```python
from build123d import *

# Parameters (mm, degrees)
CUT_EXTRUDE1_DEPTH = 4.375
CIRPATTERN1_COUNT  = 4


with BuildPart() as part:
    # Sketch1 → Revolve1 (revolve)
    with BuildSketch(Plane.XY):
        Polygon((2.1, 3), (2.1, -3), (2.6, -3), (3.125, -1.75), (2.5, -1.75), (2.5, 2.25), (3.375, 2.25), (3.375, 3), align=None)
    revolve(axis=Axis((0, 3, 0), (0, -1, 0)))

    # Sketch2 → Cut-Extrude1 (cut, symmetric)
    with BuildSketch(Plane.XY):
        Polygon((-0.249514725, 1), (0.249514725, 1), (0.625, -3), (-0.625, -3), align=None)
    cut_extrude1 = extrude(amount=CUT_EXTRUDE1_DEPTH, both=True, mode=Mode.SUBTRACT)

    # CirPattern1: Cut-Extrude1 ×4 about axis
    cirpattern1_axis = Axis((0, 3, 0), (0, 1, 0))
    for i in range(1, CIRPATTERN1_COUNT):
        add(cut_extrude1.rotate(cirpattern1_axis, i * 360 / CIRPATTERN1_COUNT), mode=Mode.SUBTRACT)


solid = part.part
```
Part model, mm, in its own coordinate system. A direction names the side the tool comes from. Round coordinates to 2 decimals unless told otherwise and drop trailing zeros. Loops run counter-clockwise (first coordinate to the right, second up) from the corner with the lowest first, then second, coordinate; pieces in that order, holes last. Notation, with made-up numbers: (-0.5, 83.5) -> (22.5, 83.5) arc R20 ccw to (22.5, 115.5) -> close; hole circle Ø7 at (18, 42.5). An arc over 180 degrees is marked (long way). Use CSV: the item, a comma, the result in double quotes. Start each with the question number.
1) Cut at B-B, the plane y = 0.5. Write the cut outline in (x, z).
2) Pull direction Y, two halves, no side cores. Call faces 1 (the flat face through (2, -1.75, -2)), 2 (the flat face through (-2, -1.75, -2)), 3 (the cylindrical face through (-0.7, 2.6, -3.3)), 4 (the flat face through (-1.6, -3, 1.7)): +Y half, -Y half, draft (parallel to the pull), parting line (faces both ways), or undercut.
3) Cut at C-C, the plane x = 0. Write the cut outline in (y, z) (3 decimals).
4) Drop flat-ended pins along their axis: P1, Ø3, axis at x = -0.5, y = -1.5, coming from the +Z side; P2, Ø3, axis at y = -2, z = 2.5, coming from the -X side; P3, Ø2, axis at x = 1.5, y = -0.5, coming from the -Z side. Give the stop position or say it passes through.
5) Cut at A-A, the plane z = 0. Write the cut outline in (x, y) (3 decimals), plus the area to 3 significant figures.
6) Which spindle directions (+Z, -Z, +X, -X, +Y, -Y) get a long thin tool onto all of the face, cutting with end or side? Do faces 5 (the cylindrical face through (2.31, 0.28, -0.96)), 6 (the flat face through (0.476, -1.416, -2.297)), 7 (the flat face through (-2.297, -1.416, -0.476)). Say none if no direction does.
7) Wall check: L1, parallel to Y at x = 2, z = -2; L2, parallel to Y at x = -2, z = 2.5; L3, parallel to X at y = -2.5, z = -0.75. Give the ranges that are in metal, low to high. Write a range as [from, to].
8) Cut at D-D, the plane y = 1.5. Write the cut outline in (x, z), plus the area to 3 significant figures.
Determined:
1,outline,"(-2.48, -0.3) arc R2.5 ccw to (-0.3, -2.48) -> (-0.3, -2.08) arc R2.1 cw to (-2.08, -0.3) -> close; (-2.48, 0.3) -> (-2.08, 0.3) arc R2.1 cw to (-0.3, 2.08) -> (-0.3, 2.48) arc R2.5 ccw to start; (0.3, -2.48) arc R2.5 ccw to (2.48, -0.3) -> (2.08, -0.3) arc R2.1 cw to (0.3, -2.08) -> close; (0.3, 2.08) arc R2.1 cw to (2.08, 0.3) -> (2.48, 0.3) arc R2.5 ccw to (0.3, 2.48) -> close"
2,face 1,"undercut"
2,face 2,"undercut"
2,face 3,"draft"
2,face 4,"-Y half"
3,outline,"(1, -2.5) -> (2.25, -2.5) -> (2.25, -3.375) -> (3, -3.375) -> (3, -2.1) -> (1, -2.1) -> close; (1, 2.1) -> (3, 2.1) -> (3, 3.375) -> (2.25, 3.375) -> (2.25, 2.5) -> (1, 2.5) -> close"
4,P1,"stops at z = 3.08"
4,P2,"stops at x = -2.95"
4,P3,"stops at z = -2.45"
5,outline,"(-3.375, 2.25) -> (-2.5, 2.25) -> (-2.5, 1) -> (-2.1, 1) -> (-2.1, 3) -> (-3.375, 3) -> close; (2.1, 1) -> (2.5, 1) -> (2.5, 2.25) -> (3.375, 2.25) -> (3.375, 3) -> (2.1, 3) -> close"
5,area,"2.91 mm2"
6,face 5,"none"
6,face 6,"+Z, -Z, -Y"
6,face 7,"+X, -X, -Y"
7,L1,"y = [-2.46, -1.75], [2.25, 3]"
7,L2,"y = [2.25, 3]"
7,L3,"x = [-2.71, -1.96], [1.96, 2.71]"
8,outline,"circle Ø5 at (0, 0); hole circle Ø4.2 at (0, 0)"
8,area,"5.78 mm2"
